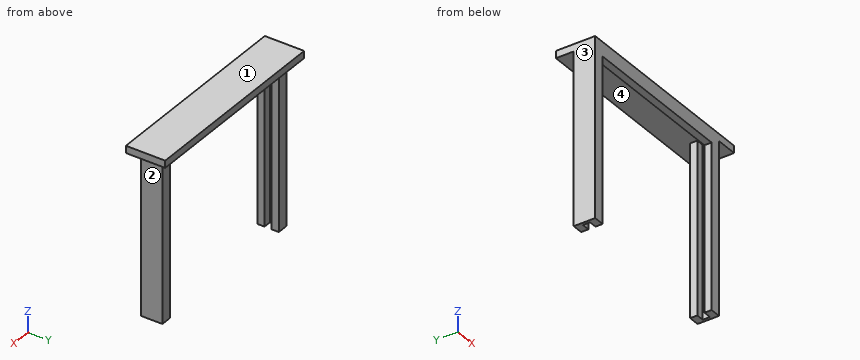
Autodesk Inventor part; units mm, degrees
ref_plane "YZ Plane" through (0, 0, 0) normal (1, 0, 0) x (0, 1, 0)
ref_plane "XZ Plane" through (0, 0, 0) normal (0, 1, 0) x (-1, 0, 0)
ref_plane "XY Plane" through (0, 0, 0) normal (0, 0, 1) x (1, 0, 0)
sketch "Sketch1" plane through (0, 0, 0) normal (0, 1, 0) x (-1, 0, 0)
  line L0 (-25, -25) -> (25, -25)
  line L1 (25, -25) -> (25, 25)
  line L2 (25, 25) -> (-25, 25)
  line L3 (-25, 25) -> (-25, -25)
  line L4 (-25, -25) -> (25, 25) construction
  line L5 (25, -25) -> (-25, 25) construction
  line L6 (25, 21) -> (-25, 21)
  line L7 (22, 21) -> (22, -25)
  line L8 (-22, 21) -> (-22, -25)
  point P0 (0, 0)
  dimension "d0" = 50
  dimension "d1" = 50
  dimension "d2" = 4
  dimension "d3" = 3
  dimension "d4" = 3
extrude "Extrusion1" add sketch "Sketch1" along normal blind 2 contours L3 L6 L8 L0 | L3 L2 L1 L6 | L7 L6 L1 L0
sketch "Sketch2" plane through (0, 2, 0) normal (0, 1, 0) x (1, 0, 0)
  line L0 (-22, 25) -> (-25, 25)
  line L1 (-25, 25) -> (-25, -25)
  line L2 (-25, -25) -> (25, -25)
  line L3 (25, -25) -> (25, 25)
  line L4 (25, 25) -> (22, 25)
  line L5 (22, 25) -> (22, -21)
  line L6 (22, -21) -> (-22, -21)
  line L7 (-22, -21) -> (-22, 25)
  line L8 (-25, -25) -> (25, -25)
  line L9 (25, -25) -> (25, -23)
  line L10 (25, -23) -> (-25, -23)
  line L11 (-25, -23) -> (-25, -25)
  point P0 (0, 0)
  dimension "d7" = 2
extrude "Extrusion2" add sketch "Sketch2" along normal blind 9 contours L10 L3 L2 L1
sketch "Sketch3" plane through (0, 2, 0) normal (0, 1, 0) x (1, 0, 0)
  line L0 (-25, -23) -> (25, -23)
  line L1 (25, -23) -> (25, 25)
  line L2 (25, 25) -> (22, 25)
  line L3 (22, 25) -> (22, -21)
  line L4 (22, -21) -> (-22, -21)
  line L5 (-22, -21) -> (-22, 25)
  line L6 (-22, 25) -> (-25, 25)
  line L7 (-25, 25) -> (-25, -23)
  line L8 (-25, -23) -> (-24.2, -23)
  line L9 (-24.2, -23) -> (-24.2, 25)
  line L10 (-24.2, 25) -> (-25, 25)
  line L11 (-25, 25) -> (-25, -23)
  line L12 (25, -23) -> (24.2, -23)
  line L13 (24.2, -23) -> (24.2, 25)
  line L14 (24.2, 25) -> (25, 25)
  line L15 (25, 25) -> (25, -23)
  point P0 (0, 0)
  dimension "d10" = 0.8
  dimension "d11" = 0.8
extrude "Extrusion3" add sketch "Sketch3" along normal blind 2 contours L7 L6 L9 L0 | L13 L2 L1 L0
sketch "Sketch4" plane through (0, 4, 0) normal (0, 1, 0) x (1, 0, 0)
  line L0 (-24.2, 25) -> (-25, 25)
  line L1 (-25, 25) -> (-25, -23)
  line L2 (-24.2, -23) -> (-25, -23)
  line L3 (-24.2, -23) -> (-24.2, 25)
  line L4 (24.2, -23) -> (24.2, 25)
  line L5 (24.2, 25) -> (22, 25)
  line L6 (22, 25) -> (22, -21)
  line L7 (22, -21) -> (-22, -21)
  line L8 (-22, -21) -> (-22, 25)
  line L9 (-22, 25) -> (-24.2, 25)
  line L10 (-24.2, 25) -> (-24.2, -23)
  line L11 (-24.2, -23) -> (24.2, -23)
  line L12 (-25, 25) -> (-22, 25)
  line L13 (-22, 25) -> (-22, -23)
  line L14 (-22, -23) -> (-25, -23)
  line L15 (-25, -23) -> (-25, 25)
  line L16 (25, -23) -> (24.2, -23)
  line L17 (25, -23) -> (25, 25)
  line L18 (25, 25) -> (24.2, 25)
  line L19 (24.2, 25) -> (24.2, -23)
  line L20 (25, -23) -> (22, -23)
  line L21 (22, -23) -> (22, 25)
  line L22 (22, 25) -> (25, 25)
  line L23 (25, 25) -> (25, -23)
  point P0 (0, 0)
extrude "Extrusion4" add sketch "Sketch4" along normal blind 2 contours L3 L2 L1 L0 | L9 L8 L13 L11 L3 | L21 L6 L5 L4 L11 | L4 L18 L17 L16
sketch "Sketch5" plane through (25, 0, 25) normal (1, 0, 0) x (0, 0, -1)
  line L0 (0, 11) -> (2, 11)
  line L1 (0, 0) -> (0, 11)
  line L2 (2, 11) -> (0, 11)
  line L3 (0, 11) -> (0, 0)
  line L4 (0, 0) -> (2, 0)
  line L5 (2, 0) -> (2, 11)
  point P0 (25, 0)
extrude "Extrusion5" add sketch "Sketch5" along normal blind 6.1
properties part number "clip_pcb-command" material "ABS Plastic"
Input: part model. Units: mm. Frame: model coordinates. Face numbers are marked on the shaded views. Round coordinates to 2 decimals unless told otherwise and drop trailing zeros. Write each loop counter-clockwise with the first axis right and the second up, starting at its lowest first coordinate (ties: lowest second). Pieces come first, ordered by that corner, then holes.
1) Contact query for flat-ended pins moving along their axis: P1, Ø0.9, axis at x = 23, z = -7, coming from the +Y side; P2, Ø2, axis at x = 1, y = 1.5, coming from the -Z side; P3, Ø1.6, axis at y = 1, z = -1.5, coming from the +X side. Output: stop coordinate, or through.
2) Cut plane C-C (x = -18). Return the cut outline in (y, z), then the cut area to 3 significant figures.
3) Ray query, L1, parallel to Y at x = 23, z = -2; L2, parallel to X at y = 3.5, z = -10; L3, parallel to X at y = 1.5, z = 8.5. Return the intervals inside material, ascending.
4) Draft query along X for the marked faces 1, 2, 3 and 4. Return one class per face: pulls with the +X half, pulls with the -X half, needs draft (parallel to the pull), parting line crosses it, or undercut.
5) Cut plane B-B (y = 3). Return the cut outline in (x, z).
6) Cut plane A-A (z = -6.5). Return the cut outline in (x, y).
7) Cut plane D-D (y = 6.75). Return the cut outline in (x, z), then the cut area to 3 significant figures.
Geometry says:
1. P1: stops at y = 6
1. P2: stops at z = 21
1. P3: stops at x = 25
2. outline: (0, 21) - (2, 21) - (2, 23) - (11, 23) - (11, 25) - (0, 25) - close
2. area: 26.0 mm2
3. L1: y = 0 to 2, 4 to 6
3. L2: x = -25 to -24.2, 24.2 to 25
3. L3: x = -25 to -22, 22 to 25
4. face 1: needs draft
4. face 2: pulls with the +X half
4. face 3: pulls with the -X half
4. face 4: undercut
5. outline: (-25, -25) - (-24.2, -25) - (-24.2, 23) - (24.2, 23) - (24.2, -25) - (25, -25) - (25, 23) - (31.1, 23) - (31.1, 25) - (-25, 25) - close
6. outline: (-25, 0) - (-22, 0) - (-22, 2) - (-24.2, 2) - (-24.2, 4) - (-22, 4) - (-22, 6) - (-25, 6) - close; (22, 0) - (25, 0) - (25, 6) - (22, 6) - (22, 4) - (24.2, 4) - (24.2, 2) - (22, 2) - close
7. outline: (-25, 23) - (31.1, 23) - (31.1, 25) - (-25, 25) - close
7. area: 112 mm2
